Autodesk Inventor part; units mm, degrees
ref_plane "YZ Plane" through (0, 0, 0) normal (1, 0, 0) x (0, 1, 0)
ref_plane "XZ Plane" through (0, 0, 0) normal (0, 1, 0) x (-1, 0, 0)
ref_plane "XY Plane" through (0, 0, 0) normal (0, 0, 1) x (1, 0, 0)
sketch "Sketch1" plane through (0, 0, 0) normal (0, 1, 0) x (-1, 0, 0)
  line L0 (0, 0) -> (-390, 0)
  line L1 (-390, 0) -> (-390, -219)
  line L2 (-390, -219) -> (0, -219)
  line L3 (0, -219) -> (0, 0)
  line L4 (-35, -38.7) -> (-255, -38.7)
  line L5 (-255, -38.7) -> (-255, -30.7)
  line L6 (-255, -30.7) -> (-35, -30.7)
  line L7 (-35, -30.7) -> (-35, -38.7)
  line L8 (-35, -97) -> (-255, -97)
  line L9 (-255, -97) -> (-255, -89)
  line L10 (-255, -89) -> (-35, -89)
  line L11 (-35, -89) -> (-35, -97)
  line L12 (68.8158, -109.5) -> (84.9045, -109.5) construction
  line L13 (-35, -180.3) -> (-255, -180.3)
  line L14 (-255, -180.3) -> (-255, -188.3)
  line L15 (-255, -188.3) -> (-35, -188.3)
  line L16 (-35, -188.3) -> (-35, -180.3)
  line L17 (-35, -122) -> (-255, -122)
  line L18 (-255, -122) -> (-255, -130)
  line L19 (-255, -130) -> (-35, -130)
  line L20 (-35, -130) -> (-35, -122)
  point P0 (0, -109.5)
  point P1 (76.8601, -109.5)
  dimension "d0" = 219
  dimension "d1" = 50.3
  dimension "d2" = 8
  dimension "d3" = 8
  dimension "d4" = 35
  dimension "d6" = 220
  dimension "d7" = 25
  dimension "d8" = 30.7
  dimension "d9" = 30.7
  dimension "d12" = 390
extrude "Extrusion1" add sketch "Sketch1" along normal blind 18
sketch "Sketch3" plane through (0, 0, 0) normal (0, -1, 0) x (1, 0, 0)
  line L0 (390, -219) -> (0, -219)
  line L1 (0, 0) -> (390, 0)
  line L2 (390, 0) -> (390, -219)
  line L3 (390, -219) -> (0, -219)
  line L4 (0, -219) -> (0, 0)
  point P0 (0, -219)
extrude "Extrusion2" add sketch "Sketch3" against normal blind 8
sketch "Sketch4" plane through (0, 18, 0) normal (0, 1, 0) x (1, 0, 0)
  line L0 (375, 15) -> (270, 15)
  line L1 (270, 15) -> (270, 204)
  line L2 (270, 204) -> (375, 204)
  line L3 (375, 204) -> (375, 15)
  line L4 (390, 0) -> (390, 219)
  line L5 (390, 219) -> (0, 219)
  line L6 (0, 0) -> (390, 0)
  line L7 (255, 130) -> (255, 122)
  line L8 (270, 204) -> (374.9963, 204) construction
  line L9 (374.9963, 204) -> (374.9963, 14.9979) construction
  line L10 (374.9963, 14.9979) -> (270, 14.9979) construction
  line L11 (270, 14.9979) -> (270, 204) construction
  point P0 (375, 109.5)
  point P1 (390, 109.5)
  dimension "d24" = 105
  dimension "d25" = 189
  dimension "d27" = 15
properties part number "dubpen-platform"
The model under review builds one solid part; all positions refer to its coordinate system, in mm. A direction names the side the tool comes from. Coordinates: 2 decimals unless noted, no trailing zeros. Write each loop counter-clockwise with the first axis right and the second up, starting at its lowest first coordinate (ties: lowest second). Pieces come first, ordered by that corner, then holes.
1) We need section A-A on y = 12.75. State the section outline as (x, z) points, then the cut area to 3 significant figures.
2) Clearance check with a flat-ended pin moving along its axis: pin 1 Ø2.5 at (x, z) = (135, -124) entering from +Y. State where the tip first meets the part, or that it passes through.
3) To check wall thickness, follow probe 1 along Z at (x, y) = (87.5, 9). State the ranges of the line that lie inside material, in increasing order.
4) We need section B-B on x = 112. State the section outline as (y, z) points, then the cut area to 3 significant figures.
5) The part is to be moulded in two halves that separate along X. For faces 1 (the face through (198, 18, -108)), 2 (the face through (390, 9, -108)), 3 (the face through (255, 13, -35)), say which applies: pulls with the +X half, pulls with the -X half, needs draft (parallel to the pull), parting line crosses it, or undercut.
6) Machinability: for faces 4 (the face through (0, 9, -111)), 5 (the face through (143, 13, -180.3)), which of the approach directions +Z, -Z, +X, -X, +Y, -Y give a long, thin tool a straight path to every point of the face, cutting with its end or side? Answer none if there is none.
Answer list:
1. outline: (0, -219) - (390, -219) - (390, 0) - (0, 0) - close; hole (35, -188.3) - (255, -188.3) - (255, -180.3) - (35, -180.3) - close; hole (35, -130) - (255, -130) - (255, -122) - (35, -122) - close; hole (35, -97) - (255, -97) - (255, -89) - (35, -89) - close; hole (35, -38.7) - (255, -38.7) - (255, -30.7) - (35, -30.7) - close
1. area: 78,400 mm2
2. pin 1: stops at y = 8
3. probe 1: z = -219 to -188.3, -180.3 to -130, -122 to -97, -89 to -38.7, -30.7 to 0
4. outline: (0, -219) - (18, -219) - (18, -188.3) - (8, -188.3) - (8, -180.3) - (18, -180.3) - (18, -130) - (8, -130) - (8, -122) - (18, -122) - (18, -97) - (8, -97) - (8, -89) - (18, -89) - (18, -38.7) - (8, -38.7) - (8, -30.7) - (18, -30.7) - (18, 0) - (0, 0) - close
4. area: 3,620 mm2
5. face 1: needs draft
5. face 2: pulls with the +X half
5. face 3: undercut
6. face 4: +Z, -Z, -X, +Y, -Y
6. face 5: +Y
